from build123d import *

# Parameters (mm, degrees)
ESQUISSE1_W             = 12
ESQUISSE1_H             = 12
BOSS_EXTRU_1_DEPTH      = 0.5
ESQUISSE2_W             = 11.2
ESQUISSE2_H             = 11.2
BOSS_EXTRU_2_DEPTH      = 1
CONG_1_R                = 0.3
ESQUISSE3_R             = 0.75
ENL_V_MAT_EXTRU_1_DEPTH = 0.01


with BuildPart() as part:
    # Esquisse1 → Boss.-Extru.1 (new body)
    with BuildSketch(Plane.XY):
        with Locations((6, -6)):
            Rectangle(ESQUISSE1_W, ESQUISSE1_H)
    extrude(amount=BOSS_EXTRU_1_DEPTH)

    # Esquisse2 → Boss.-Extru.2 (add)
    with BuildSketch(Plane.XY.offset(0.5)):
        with Locations((6, -6)):
            Rectangle(ESQUISSE2_W, ESQUISSE2_H)
    extrude(amount=BOSS_EXTRU_2_DEPTH)

    # Congé1
    cong_1_edges = [part.edges().sort_by_distance(p)[0] for p in [
        (0.4, -0.4, 1),
        (0.4, -11.6, 1),
        (11.6, -11.6, 1),
        (11.6, -0.4, 1),
    ]]
    fillet(cong_1_edges, radius=CONG_1_R)

    # Esquisse3 → Enlèv. mat.-Extru.1 (cut)
    with BuildSketch(Plane.XY.offset(1.5)):
        with Locations((10, -10)):
            Circle(ESQUISSE3_R)
    extrude(amount=-ENL_V_MAT_EXTRU_1_DEPTH, mode=Mode.SUBTRACT)


solid = part.part
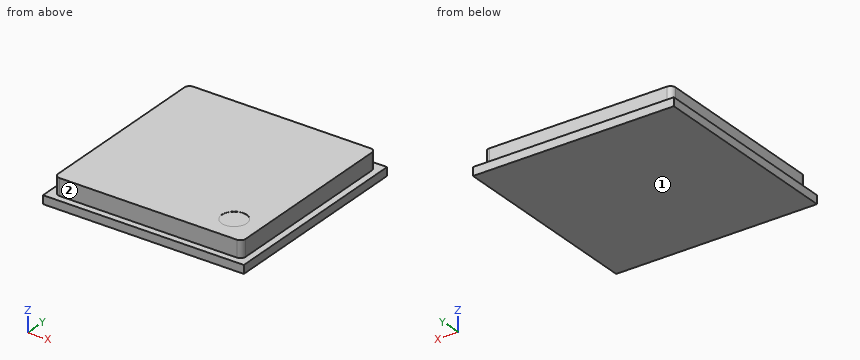
The model under review builds one solid part; all positions refer to its coordinate system, in mm. Face numbers are marked on the shaded views. A direction names the side the tool comes from. Round coordinates to 2 decimals unless told otherwise and drop trailing zeros. Write each loop counter-clockwise with the first axis right and the second up, starting at its lowest first coordinate (ties: lowest second). Pieces come first, ordered by that corner, then holes. Notation, with made-up numbers: M 34,-15 L 79,-15 A27 ccw 79,22 Z; hole C 61.5,51.5 d8. An arc over 180 degrees is marked long. Use a Markdown table: item, result. Add a question column.
Q1. We need section D-D, the plane y = -1.25. State the section outline as (x, z) points.
Q2. To check wall thickness, follow line 1 (Y direction, x = 7, z = 0.55); line 2 (X direction, y = -10.25, z = 1.25); line 3 (X direction, y = -11.5, z = 0.6). State the ranges of each line that lie inside material, in increasing order.
Q3. Insertion check: pin 1 (0.8 mm diameter, centred on y = -6, z = 1, fed in from +X). The pin has a flat end and moves straight along its axis. Give the tip position at first contact, or say it passes through.
Q4. Machinability: for the marked faces 1 and 2, which of the approach directions +Z, -Z, +X, -X, +Y, -Y give a long, thin tool a straight path to every point of the face, cutting with its end or side? Answer none if there is none.
Q5. We need section B-B, the plane z = 1.2. State the section outline as (x, y) points.
Findings below:
| question | item | result |
|---|---|---|
| 1 | outline | M 0,0 L 12,0 L 12,0.5 L 11.6,0.5 L 11.6,1.5 L 0.4,1.5 L 0.4,0.5 L 0,0.5 Z |
| 2 | line 1 | y = -11.6 to -0.4 |
| 2 | line 2 | x = 0.4 to 11.6 |
| 2 | line 3 | x = 0.48 to 11.52 |
| 3 | pin 1 | stops at x = 11.6 |
| 4 | face 1 | -Z, +X, -X, +Y, -Y |
| 4 | face 2 | +Z, +X, -X, -Y |
| 5 | outline | M 0.4,-11.3 A0.3 ccw 0.7,-11.6 L 11.3,-11.6 A0.3 ccw 11.6,-11.3 L 11.6,-0.7 A0.3 ccw 11.3,-0.4 L 0.7,-0.4 A0.3 ccw 0.4,-0.7 Z |
